Could you check a few things on this model? Use its own coordinates, in mm. Face numbers are marked on the shaded views. A direction names the side the tool comes from. Give positions to 0.01 mm unless a question says otherwise; leave off trailing zeros. Order: outer loops, then holes, each group sorted by start corner. A loop starts at its lowest first (then second) coordinate and runs counter-clockwise, first axis right, second up. Notation, with made-up numbers: (-34, -29) - (17, -29) arc R8 cw to (17, -24) - close; hole circle Ø2 at (-24, 72.25). An arc over 180 degrees is marked (long way). One line per question, with ' | ' between items. Start each with the question number.
1. Imagine slicing it at D-D (z = -8.5). Please give me the cut outline in (x, y), and give its area (3 significant figures).
2. Imagine slicing it at A-A (x = 4.75). Please give me the cut outline in (y, z).
3. If we mould it in two halves opening along Z, with no side actions, what happens to the marked faces 1, 2, 3 and 4? For each: released by +Z, released by -Z, zero draft, split by the parting line, or undercut.
4. Imagine slicing it at C-C (y = 39.5). Please give me the cut outline in (x, z).
5. For P1, Ø3.5, axis at y = 61, z = 13.7, coming from the +X side; P2, Ø10, axis at y = 15.5, z = 3, coming from the -X side, each with a flat end and sliding along its axis, tell me the tip position at first contact or that it passes through.
6. Imagine slicing it at B-B (z = 13.7). Please give me the cut outline in (x, y).
7. I need wall thicknesses on probe 1 along Y at (x, z) = (4.4, 13.7); probe 2 along Y at (x, z) = (2.7, -16.3); probe 3 along Y at (x, z) = (1.8, 3.5). Which ranges of each line are inside material? Lowest first, please. Write a range as from..to.
8. Which directions (+Z, -Z, +X, -X, +Y, -Y) give clear straight access to the entire face, cutting with the end or side of a thin tool? Please do the marked faces 5, 6, 7 and 8.
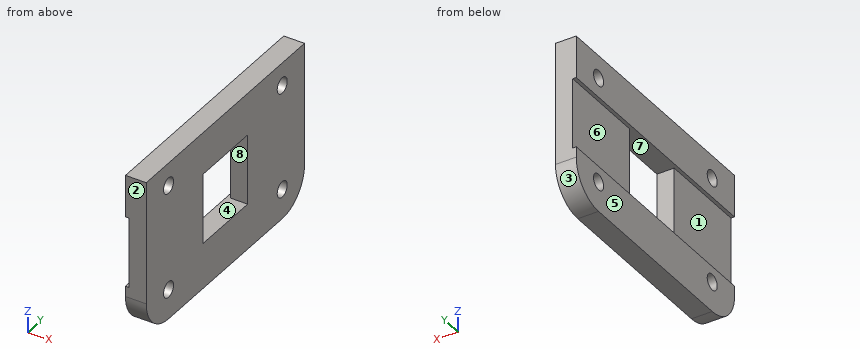
```python
from build123d import *

# Parameters (mm, degrees)
SKETCH1_W           = 5.9
SKETCH1_H           = 45
BOSS_EXTRUDE1_DEPTH = 71
CUT_EXTRUDE2_REACH  = 73
SKETCH3_W           = 1
SKETCH3_H           = 20
FILLET1_R           = 10
CUT_EXTRUDE3_REACH  = 7.9
SKETCH4_R           = 2.25
CUT_EXTRUDE4_REACH  = 7.9
SKETCH5_W           = 20
SKETCH5_H           = 20


with BuildPart() as part:
    # Sketch1 → Boss-Extrude1 (new body)
    with BuildSketch(Plane(origin=(0, 0, 0), x_dir=(1, 0, 0), z_dir=(0, 1, 0))):
        with Locations((2.95, 2.3)):
            Rectangle(SKETCH1_W, SKETCH1_H)
    extrude(amount=BOSS_EXTRUDE1_DEPTH)

    # Sketch3 → Cut-Extrude2 (cut, up to next)
    with BuildSketch(Plane.XZ, mode=Mode.PRIVATE) as cut_extrude2_sk1:
        with Locations((0.5, -1.8)):
            Rectangle(SKETCH3_W, SKETCH3_H)
    cut_extrude2_tool1 = extrude(cut_extrude2_sk1.sketch, amount=-CUT_EXTRUDE2_REACH, mode=Mode.PRIVATE) & part.part
    add(cut_extrude2_tool1.solids().sort_by_distance((0.5, 0, -1.8))[0], mode=Mode.SUBTRACT)

    # Fillet1
    fillet1_edges = [part.edges().sort_by_distance(p)[0] for p in [
        (2.95, 71, -24.8),
        (2.95, 0, -24.8),
    ]]
    fillet(fillet1_edges, radius=FILLET1_R)

    # Sketch4 → Cut-Extrude3 (cut, up to next)
    with BuildSketch(Plane(origin=(5.9, 0, 0), x_dir=(0, 0, -1), z_dir=(1, 0, 0)), mode=Mode.PRIVATE) as cut_extrude3_sk1:
        with Locations((-13.7, 61)):
            Circle(SKETCH4_R)
    cut_extrude3_tool1 = extrude(cut_extrude3_sk1.sketch, amount=-CUT_EXTRUDE3_REACH, mode=Mode.PRIVATE) & part.part
    add(cut_extrude3_tool1.solids().sort_by_distance((5.9, 61, 13.7))[0], mode=Mode.SUBTRACT)
    # Sketch4 → Cut-Extrude3 (cut, up to next)
    with BuildSketch(Plane(origin=(5.9, 0, 0), x_dir=(0, 0, -1), z_dir=(1, 0, 0)), mode=Mode.PRIVATE) as cut_extrude3_sk2:
        with Locations((-13.7, 10)):
            Circle(SKETCH4_R)
    cut_extrude3_tool2 = extrude(cut_extrude3_sk2.sketch, amount=-CUT_EXTRUDE3_REACH, mode=Mode.PRIVATE) & part.part
    add(cut_extrude3_tool2.solids().sort_by_distance((5.9, 10, 13.7))[0], mode=Mode.SUBTRACT)
    # Sketch4 → Cut-Extrude3 (cut, up to next)
    with BuildSketch(Plane(origin=(5.9, 0, 0), x_dir=(0, 0, -1), z_dir=(1, 0, 0)), mode=Mode.PRIVATE) as cut_extrude3_sk3:
        with Locations((16.3, 10)):
            Circle(SKETCH4_R)
    cut_extrude3_tool3 = extrude(cut_extrude3_sk3.sketch, amount=-CUT_EXTRUDE3_REACH, mode=Mode.PRIVATE) & part.part
    add(cut_extrude3_tool3.solids().sort_by_distance((5.9, 10, -16.3))[0], mode=Mode.SUBTRACT)
    # Sketch4 → Cut-Extrude3 (cut, up to next)
    with BuildSketch(Plane(origin=(5.9, 0, 0), x_dir=(0, 0, -1), z_dir=(1, 0, 0)), mode=Mode.PRIVATE) as cut_extrude3_sk4:
        with Locations((16.3, 61)):
            Circle(SKETCH4_R)
    cut_extrude3_tool4 = extrude(cut_extrude3_sk4.sketch, amount=-CUT_EXTRUDE3_REACH, mode=Mode.PRIVATE) & part.part
    add(cut_extrude3_tool4.solids().sort_by_distance((5.9, 61, -16.3))[0], mode=Mode.SUBTRACT)

    # Sketch5 → Cut-Extrude4 (cut, up to next)
    with BuildSketch(Plane(origin=(5.9, 0, 0), x_dir=(0, 0, -1), z_dir=(1, 0, 0)), mode=Mode.PRIVATE) as cut_extrude4_sk1:
        with Locations((1.8, 35.5)):
            Rectangle(SKETCH5_W, SKETCH5_H)
    cut_extrude4_tool1 = extrude(cut_extrude4_sk1.sketch, amount=-CUT_EXTRUDE4_REACH, mode=Mode.PRIVATE) & part.part
    add(cut_extrude4_tool1.solids().sort_by_distance((5.9, 35.5, -1.8))[0], mode=Mode.SUBTRACT)


solid = part.part
```
Results found:
1) outline: (1, 0) - (5.9, 0) - (5.9, 25.5) - (1, 25.5) - close; (1, 45.5) - (5.9, 45.5) - (5.9, 71) - (1, 71) - close | area: 250 mm2
2) outline: (0, -14.8) arc R10 ccw to (10, -24.8) - (61, -24.8) arc R10 ccw to (71, -14.8) - (71, 20.2) - (0, 20.2) - close; hole circle Ø4.5 at (10, -16.3); hole circle Ø4.5 at (10, 13.7); hole (25.5, -11.8) - (45.5, -11.8) - (45.5, 8.2) - (25.5, 8.2) - close; hole circle Ø4.5 at (61, -16.3); hole circle Ø4.5 at (61, 13.7)
3) face 1: undercut | face 2: zero draft | face 3: released by -Z | face 4: undercut
4) outline: (0, -24.8) - (5.9, -24.8) - (5.9, -11.8) - (0, -11.8) - close; (0, 8.2) - (5.9, 8.2) - (5.9, 20.2) - (0, 20.2) - close
5) P1: passes through | P2: stops at x = 1
6) outline: (0, 0) - (5.9, 0) - (5.9, 7.75) - (0, 7.75) - close; (0, 12.25) - (5.9, 12.25) - (5.9, 58.75) - (0, 58.75) - close; (0, 63.25) - (5.9, 63.25) - (5.9, 71) - (0, 71) - close
7) probe 1: y = 0..7.75, 12.25..58.75, 63.25..71 | probe 2: y = 0.11..7.75, 12.25..58.75, 63.25..70.89 | probe 3: y = 0..25.5, 45.5..71
8) face 5: +Z, -Z, -X, +Y, -Y | face 6: -X, +Y, -Y | face 7: -X | face 8: +X, -X
